Here's how the part is built. I have some questions about the finished solid (model axes, mm). Coordinates: 2 decimals unless noted, no trailing zeros. Write each loop counter-clockwise with the first axis right and the second up, starting at its lowest first coordinate (ties: lowest second). Pieces come first, ordered by that corner, then holes.
(1) Please list where these lines run through material, in increasing order: probe 1 along Y at (x, z) = (-42.7, -2); probe 2 along X at (y, z) = (2, -1.3); probe 3 along Y at (x, z) = (-65.5, -0.45).
(2) Imagine slicing it at B-B, the plane y = 0. List the corners of the cut face in (x, z) for me, plus the area to 3 significant figures.
(3) Imagine slicing it at A-A, the plane x = -67.7. List the corners of the cut face in (y, z) for me.
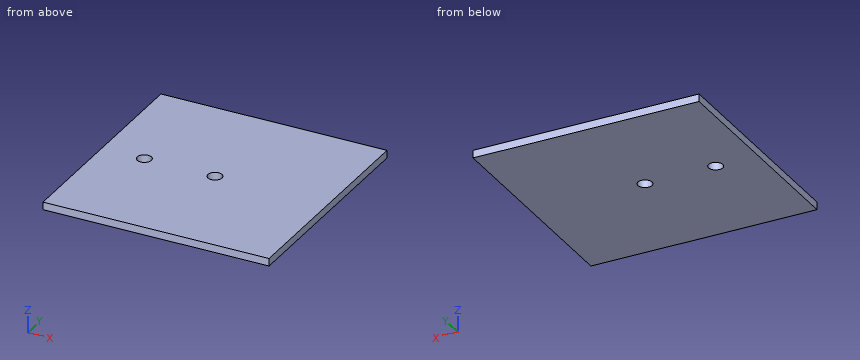
```python
from build123d import *

# Parameters (mm, degrees)
CROQUIS1_W              = 80
CROQUIS1_H              = 80
SALIENTE_EXTRUIR2_DEPTH = 2.7
CROQUIS2_R              = 2.5
CORTAR_EXTRUIR1_DEPTH   = 2.7


with BuildPart() as part:
    # Croquis1 → Saliente-Extruir2 (new body)
    with BuildSketch(Plane.XY):
        with Locations((-42.7, 0)):
            Rectangle(CROQUIS1_W, CROQUIS1_H)
    extrude(amount=-SALIENTE_EXTRUIR2_DEPTH)

    # Croquis2 → Cortar-Extruir1 (cut)
    with BuildSketch(Plane(origin=(0, 0, -2.7), x_dir=(-1, 0, 0), z_dir=(0, 0, -1))):
        with Locations((67.7, 0)):
            Circle(CROQUIS2_R)
        with Locations((42.7, 0)):
            Circle(CROQUIS2_R)
    extrude(amount=-CORTAR_EXTRUIR1_DEPTH, mode=Mode.SUBTRACT)


solid = part.part
```
Recorded:
1. probe 1: y = -40 to -2.5, 2.5 to 40
1. probe 2: x = -82.7 to -69.2, -66.2 to -44.2, -41.2 to -2.7
1. probe 3: y = -40 to -1.19, 1.19 to 40
2. outline: (-82.7, -2.7) - (-70.2, -2.7) - (-70.2, 0) - (-82.7, 0) - close; (-65.2, -2.7) - (-45.2, -2.7) - (-45.2, 0) - (-65.2, 0) - close; (-40.2, -2.7) - (-2.7, -2.7) - (-2.7, 0) - (-40.2, 0) - close
2. area: 189 mm2
3. outline: (-40, -2.7) - (-2.5, -2.7) - (-2.5, 0) - (-40, 0) - close; (2.5, -2.7) - (40, -2.7) - (40, 0) - (2.5, 0) - close
